Source: CAD feature listing. Evaluate the final solid. Frame: model axes, mm. Coordinates: 2 decimals unless noted, no trailing zeros. Write each loop counter-clockwise with the first axis right and the second up, starting at its lowest first coordinate (ties: lowest second). Pieces come first, ordered by that corner, then holes. Notation, with made-up numbers: (72, 2.5) -> (77, 2.5) arc R29 ccw to (77, 36.5) -> close; hole circle Ø3 at (-32.5, 74). An arc over 180 degrees is marked (long way). One line per item, written item: value. Start each with the question number.
1. First-contact query: P1, Ø8, axis at x = 42.5, y = 0, coming from the -Z side. Flat tip, straight axial feed; report the tip coordinate or a pass-through.
2. Section query D-D, the plane y = -5.25. Output: boundary loops of the cut face in (x, z), and give its area (3 significant figures).
3. Section query C-C, the plane z = 0.7. Output: boundary loops of the cut face in (x, y).
4. Section query A-A, the plane y = 0. Output: boundary loops of the cut face in (x, z).
5. Mould query, pull axis X, two halves, no side actions, for faces 1 (the cylindrical face through (44.81, -0.96, 1.48)), 2 (the cylindrical face through (50, 0, 1)), 3 (the flat face through (-1, 3, 3)). Classes: released by +X, released by -X, zero draft, split by the parting line, or undercut.
6. Line query: line 1 (Y direction, x = 0, z = 1.55); line 2 (X direction, y = 0.75, z = 1.15); line 3 (Y direction, x = -42.5, z = 1.35). Output: solid intervals per line, ascending.
7. Section query B-B, the plane x = 0. Output: boundary loops of the cut face in (y, z).
from build123d import *

# Parameters (mm, degrees)
SKETCH_1_R      = 4
SKETCH_1_R_2    = 2.5
EXTRUDE_1_DEPTH = 3


with BuildPart() as part:
    # 草图1 → 凸台-拉伸1 (new body)
    with BuildSketch(Plane.XY):
        with BuildLine():
            Line((-42.5, -7.5), (42.5, -7.5))
            ThreePointArc((42.5, -7.5), (50, 0), (42.5, 7.5))
            Line((42.5, 7.5), (-42.5, 7.5))
            ThreePointArc((-42.5, 7.5), (-50, 0), (-42.5, -7.5))
        make_face()
        with Locations((-42.5, 0)):
            Circle(SKETCH_1_R, mode=Mode.SUBTRACT)
        with Locations((42.5, 0)):
            Circle(SKETCH_1_R_2, mode=Mode.SUBTRACT)
        Circle(SKETCH_1_R_2, mode=Mode.SUBTRACT)
    extrude(amount=EXTRUDE_1_DEPTH)


solid = part.part
Computed values:
1. P1: stops at z = 0
2. outline: (-47.86, 0) -> (47.86, 0) -> (47.86, 3) -> (-47.86, 3) -> close
2. area: 287 mm²
3. outline: (-42.5, -7.5) -> (42.5, -7.5) arc R7.5 ccw to (42.5, 7.5) -> (-42.5, 7.5) arc R7.5 ccw to start; hole circle Ø8 at (-42.5, 0); hole circle Ø5 at (0, 0); hole circle Ø5 at (42.5, 0)
4. outline: (-50, 0) -> (-46.5, 0) -> (-46.5, 3) -> (-50, 3) -> close; (-38.5, 0) -> (-2.5, 0) -> (-2.5, 3) -> (-38.5, 3) -> close; (2.5, 0) -> (40, 0) -> (40, 3) -> (2.5, 3) -> close; (45, 0) -> (50, 0) -> (50, 3) -> (45, 3) -> close
5. face 1: undercut
5. face 2: released by +X
5. face 3: zero draft
6. line 1: y = -7.5 to -2.5, 2.5 to 7.5
6. line 2: x = -49.96 to -46.43, -38.57 to -2.38, 2.38 to 40.12, 44.88 to 49.96
6. line 3: y = -7.5 to -4, 4 to 7.5
7. outline: (-7.5, 0) -> (-2.5, 0) -> (-2.5, 3) -> (-7.5, 3) -> close; (2.5, 0) -> (7.5, 0) -> (7.5, 3) -> (2.5, 3) -> close
